```python
from build123d import *

# Parameters (mm, degrees)
F0_R     = 14.037326
F1_DEPTH = 13.208


with BuildPart() as f1:
    # F0 (on Top) → F1 (new body)
    with BuildSketch(Plane.XY):
        with BuildLine():
            ThreePointArc((24.666504, -3.280848), (24.82937, -1.644016), (24.883737, 0))
            ThreePointArc((24.883737, 0), (24.82937, 1.644016), (24.666504, 3.280848))
            ThreePointArc((24.666504, 3.280848), (24.035844, 6.440385), (23.002243, 9.491954))
            ThreePointArc((23.002243, 9.491954), (21.549949, 12.441869), (19.721395, 15.17455))
            ThreePointArc((19.721395, 15.17455), (17.595459, 17.595459), (15.17455, 19.721395))
            ThreePointArc((15.17455, 19.721395), (12.441869, 21.549949), (9.491954, 23.002243))
            ThreePointArc((9.491954, 23.002243), (6.440385, 24.035844), (3.280848, 24.666504))
            ThreePointArc((3.280848, 24.666504), (0, 24.883737), (-3.280848, 24.666504))
            ThreePointArc((-3.280848, 24.666504), (-6.440385, 24.035844), (-9.491954, 23.002243))
            ThreePointArc((-9.491954, 23.002243), (-12.441869, 21.549949), (-15.17455, 19.721395))
            ThreePointArc((-15.17455, 19.721395), (-17.595459, 17.595459), (-19.721395, 15.17455))
            ThreePointArc((-19.721395, 15.17455), (-21.549949, 12.441869), (-23.002243, 9.491954))
            ThreePointArc((-23.002243, 9.491954), (-24.035844, 6.440385), (-24.666504, 3.280848))
            ThreePointArc((-24.666504, 3.280848), (-24.883737, 0), (-24.666504, -3.280848))
            ThreePointArc((-24.666504, -3.280848), (-24.035844, -6.440385), (-23.002243, -9.491954))
            ThreePointArc((-23.002243, -9.491954), (-21.549949, -12.441869), (-19.721395, -15.17455))
            ThreePointArc((-19.721395, -15.17455), (-17.595459, -17.595459), (-15.17455, -19.721395))
            ThreePointArc((-15.17455, -19.721395), (-12.441869, -21.549949), (-9.491954, -23.002243))
            ThreePointArc((-9.491954, -23.002243), (-6.440385, -24.035844), (-3.280848, -24.666504))
            ThreePointArc((-3.280848, -24.666504), (0, -24.883737), (3.280848, -24.666504))
            ThreePointArc((3.280848, -24.666504), (6.440385, -24.035844), (9.491954, -23.002243))
            ThreePointArc((9.491954, -23.002243), (12.441869, -21.549949), (15.17455, -19.721395))
            ThreePointArc((15.17455, -19.721395), (17.595459, -17.595459), (19.721395, -15.17455))
            ThreePointArc((19.721395, -15.17455), (21.549949, -12.441869), (23.002243, -9.491954))
            ThreePointArc((23.002243, -9.491954), (24.035844, -6.440385), (24.666504, -3.280848))
        make_face()
        Circle(F0_R, mode=Mode.SUBTRACT)
        with BuildLine():
            ThreePointArc((24.666504, 3.280848), (24.82937, 1.644016), (24.883737, 0))
            ThreePointArc((24.883737, 0), (24.82937, -1.644016), (24.666504, -3.280848))
            Line((24.666504, -3.280848), (31.178985, -1.803033))
            Line((31.178985, -1.803033), (31.178985, 0))
            Line((31.178985, 0), (31.178985, 1.803033))
            Line((31.178985, 1.803033), (24.666504, 3.280848))
        make_face()
        with BuildLine():
            ThreePointArc((19.721395, 15.17455), (21.549949, 12.441869), (23.002243, 9.491954))
            Line((23.002243, 9.491954), (27.903309, 14.02802))
            Line((27.903309, 14.02802), (27.001793, 15.589492))
            Line((27.001793, 15.589492), (26.100276, 17.150965))
            Line((26.100276, 17.150965), (19.721395, 15.17455))
        make_face()
        with BuildLine():
            Line((27.903309, -14.02802), (23.002243, -9.491954))
            ThreePointArc((23.002243, -9.491954), (21.549949, -12.441869), (19.721395, -15.17455))
            Line((19.721395, -15.17455), (26.100276, -17.150965))
            Line((26.100276, -17.150965), (27.001793, -15.589492))
            Line((27.001793, -15.589492), (27.903309, -14.02802))
        make_face()
        with BuildLine():
            ThreePointArc((9.491954, 23.002243), (12.441869, 21.549949), (15.17455, 19.721395))
            Line((15.17455, 19.721395), (17.150965, 26.100276))
            Line((17.150965, 26.100276), (15.589492, 27.001793))
            Line((15.589492, 27.001793), (14.02802, 27.903309))
            Line((14.02802, 27.903309), (9.491954, 23.002243))
        make_face()
        with BuildLine():
            Line((17.150965, -26.100276), (15.17455, -19.721395))
            ThreePointArc((15.17455, -19.721395), (12.441869, -21.549949), (9.491954, -23.002243))
            Line((9.491954, -23.002243), (14.02802, -27.903309))
            Line((14.02802, -27.903309), (15.589492, -27.001793))
            Line((15.589492, -27.001793), (17.150965, -26.100276))
        make_face()
        with BuildLine():
            ThreePointArc((-3.280848, 24.666504), (0, 24.883737), (3.280848, 24.666504))
            Line((3.280848, 24.666504), (1.803033, 31.178985))
            Line((1.803033, 31.178985), (0, 31.178985))
            Line((0, 31.178985), (-1.803033, 31.178985))
            Line((-1.803033, 31.178985), (-3.280848, 24.666504))
        make_face()
        with BuildLine():
            Line((1.803033, -31.178985), (3.280848, -24.666504))
            ThreePointArc((3.280848, -24.666504), (0, -24.883737), (-3.280848, -24.666504))
            Line((-3.280848, -24.666504), (-1.803033, -31.178985))
            Line((-1.803033, -31.178985), (0, -31.178985))
            Line((0, -31.178985), (1.803033, -31.178985))
        make_face()
        with BuildLine():
            ThreePointArc((-15.17455, 19.721395), (-12.441869, 21.549949), (-9.491954, 23.002243))
            Line((-9.491954, 23.002243), (-14.02802, 27.903309))
            Line((-14.02802, 27.903309), (-15.589492, 27.001793))
            Line((-15.589492, 27.001793), (-17.150965, 26.100276))
            Line((-17.150965, 26.100276), (-15.17455, 19.721395))
        make_face()
        with BuildLine():
            Line((-14.02802, -27.903309), (-9.491954, -23.002243))
            ThreePointArc((-9.491954, -23.002243), (-12.441869, -21.549949), (-15.17455, -19.721395))
            Line((-15.17455, -19.721395), (-17.150965, -26.100276))
            Line((-17.150965, -26.100276), (-15.589492, -27.001793))
            Line((-15.589492, -27.001793), (-14.02802, -27.903309))
        make_face()
        with BuildLine():
            ThreePointArc((-23.002243, 9.491954), (-21.549949, 12.441869), (-19.721395, 15.17455))
            Line((-19.721395, 15.17455), (-26.100276, 17.150965))
            Line((-26.100276, 17.150965), (-27.001793, 15.589492))
            Line((-27.001793, 15.589492), (-27.903309, 14.02802))
            Line((-27.903309, 14.02802), (-23.002243, 9.491954))
        make_face()
        with BuildLine():
            Line((-26.100276, -17.150965), (-19.721395, -15.17455))
            ThreePointArc((-19.721395, -15.17455), (-21.549949, -12.441869), (-23.002243, -9.491954))
            Line((-23.002243, -9.491954), (-27.903309, -14.02802))
            Line((-27.903309, -14.02802), (-27.001793, -15.589492))
            Line((-27.001793, -15.589492), (-26.100276, -17.150965))
        make_face()
        with BuildLine():
            ThreePointArc((-24.666504, -3.280848), (-24.883737, 0), (-24.666504, 3.280848))
            Line((-24.666504, 3.280848), (-31.178985, 1.803033))
            Line((-31.178985, 1.803033), (-31.178985, 0))
            Line((-31.178985, 0), (-31.178985, -1.803033))
            Line((-31.178985, -1.803033), (-24.666504, -3.280848))
        make_face()
    extrude(amount=F1_DEPTH)


solid = f1.part
```
Source: CAD feature listing. Evaluate the final solid. Frame: model axes, mm. A direction names the side the tool comes from. Round coordinates to 2 decimals unless told otherwise and drop trailing zeros. Loops run counter-clockwise (first coordinate to the right, second up) from the corner with the lowest first, then second, coordinate; pieces in that order, holes last. Notation, with made-up numbers: M -7.75,34 L 26.25,34 A25 ccw 26.25,53 Z; hole C -8.75,24 d7. An arc over 180 degrees is marked long. Use a Markdown table: item, result. Add a question column.
1. Mould query, pull axis X, two halves, no side actions, for faces 1 (the flat face through (-16.15, -22.87, 6.51)), 2 (the cylindrical face through (17.63, 17.56, 6.51)), 3 (the cylindrical face through (24.047, 6.397, 6.512)). Classes: pulls with the +X half, pulls with the -X half, needs draft (parallel to the pull), parting line crosses it, or undercut.
2. Line query: line 1 (Y direction, x = 0, z = 5.75); line 2 (Y direction, x = 27, z = 11.25); line 3 (Y direction, x = 26.5, z = 10.75). Output: solid intervals per line, ascending.
3. Section query D-D on y = -22. Return the cut outline in (x, z), then the cut area to 4 significant figures.
4. Section query A-A on x = 0. Return the cut outline in (y, z).
5. Contact query for flat-ended pins moving along their axis: P1, Ø2, axis at x = 17, y = -17, coming from the -Z side; P2, Ø1.5, axis at x = -20.5, y = 17.5, coming from the -Z side; P3, Ø6, axis at x = 13.5, z = 8.5, coming from the +Y side; P4, Ø5, axis at x = 23.5, z = 5.5, coming from the -Y side. Output: stop coordinate, or through.
6. Section query C-C on y = 20.5. Return the cut outline in (x, z).
7. Reachability of faces 4 (the flat face through (11.792, 25.487, 6.512)), 5 (the flat face through (27.97, 2.53, 6.51)), 6 (the cylindrical face through (-6.484, -24.024, 6.512)), 7 (the cylindrical face through (-24.047, -6.397, 6.512)) from +Z, -Z, +X, -X, +Y, -Y: full face, straight path, thin tool, end or side. Return the list, or none.
Reported:
| question | item | result |
|---|---|---|
| 1 | face 1 | pulls with the -X half |
| 1 | face 2 | undercut |
| 1 | face 3 | pulls with the +X half |
| 2 | line 1 | y = -31.18 to -14.04, 14.04 to 31.18 |
| 2 | line 2 | y = -15.59 to -13.19, -2.75 to 2.75, 13.19 to 15.59 |
| 2 | line 3 | y = -16.46 to -12.73, -2.86 to 2.86, 12.73 to 16.46 |
| 3 | outline | M -15.88,0 L 15.88,0 L 15.88,13.21 L -15.88,13.21 Z |
| 3 | area | 419.5 mm² |
| 4 | outline | M -31.18,0 L -14.04,0 L -14.04,13.21 L -31.18,13.21 Z; M 14.04,0 L 31.18,0 L 31.18,13.21 L 14.04,13.21 Z |
| 5 | P1 | stops at z = 0 |
| 5 | P2 | passes through |
| 5 | P3 | stops at y = 27.9 |
| 5 | P4 | stops at y = -17.12 |
| 6 | outline | M -15.42,0 L 15.42,0 L 15.42,13.21 L -15.42,13.21 Z |
| 7 | face 4 | +Z, -Z, +Y |
| 7 | face 5 | +Z, -Z, +X |
| 7 | face 6 | +Z, -Z, -Y |
| 7 | face 7 | +Z, -Z, -X |
